Autodesk Inventor part; units mm, degrees
ref_plane "Work Plane2" through (-27.2, 5.425, 1.675) normal (1, 0, 0) x (0, 1, 0)
ref_plane "Work Plane3" through (-22.5, 37.5, -3) normal (-1, 0, 0) x (0, 0, 1)
ref_plane "YZ Plane" through (0, 0, 0) normal (1, 0, 0) x (0, 1, 0)
ref_plane "Work Plane1" through (-73.7, 19.125, 15.375) normal (-1, 0, 0) x (0, 1, 0)
sketch "Sketch1" plane through (-73.7, 19.125, 15.375) normal (-1, 0, 0) x (0, 1, 0)
  line L0 (18.375, 18.375) -> (-92.625, 18.375)
  line L1 (-92.625, 18.375) -> (-92.625, 15.375)
  line L2 (18.375, 15.375) -> (-92.625, 15.375)
  line L3 (18.375, 18.375) -> (18.375, 15.375)
  line L4 (11, 1.5) -> (11.5, 1.5)
  line L5 (11.5, 1.5) -> (11.5, -1.5)
  line L6 (11.5, -1.5) -> (11, -1.5)
  line L7 (11, -1.5) -> (11, 1.5)
  line L8 (-11.5, -1.5) -> (-12, -1.5)
  line L9 (-12, -1.5) -> (-12, 1.5)
  line L10 (-12, 1.5) -> (-11.5, 1.5)
  line L11 (-11.5, 1.5) -> (-11.5, -1.5)
  circle A0 centre (0, 0) radius 5
  circle A1 centre (0, 0) radius 13.7
  line L12 (18.375, 15.375) -> (-18.1, 15.375)
  line L13 (-18.1, 15.375) -> (-18.1, -4)
  line L14 (-18.1, -4) -> (18.375, -4)
  line L15 (18.375, -4) -> (18.375, 15.375)
  point P0 (-19.125, 15.375)
  point P1 (-13.7, 0)
  point P2 (13.7, 0)
  point P3 (-18.1, 15.375)
  point P4 (-13.1031, -4)
  point P5 (13.1031, -4)
  dimension "d0" = 4
  dimension "d2" = 15.375
  dimension "d3" = 15.375
  dimension "d4" = 4.675
  dimension "d5" = 4.4
ref_plane "Work Plane2" through (-27.2, 5.425, 1.675) normal (1, 0, 0) x (0, 1, 0)
extrude "Extrusion1" add sketch "Sketch1" against normal up to surface (46.5 mm away) contours L15 L14 A1 L13 L2
sketch "Sketch2" plane through (-27.2, 19.125, 15.375) normal (1, 0, 0) x (0, 0, -1)
  circle A0 centre (0, -8) radius 1.0564
  circle A1 centre (0, 8) radius 1.0564
  circle A2 centre (0, 0) radius 5
  circle A3 centre (0, 0) radius 13.7
  line L0 (18.375, 18.375) -> (18.375, -91.625)
  arc A4 (1.3629, -5.6821) -> (1.478, -3.5703) centre (-3.2424, -4.3721) ccw
  arc A5 (1.478, -3.5703) -> (2.0183, -3.2951) centre (0, 0) ccw
  arc A6 (2.0183, -3.2951) -> (3.794, -4.444) centre (5.443, 0.0511) ccw
  arc A7 (3.794, -4.444) -> (4.4425, -3.7958) centre (0, 0) ccw
  arc A8 (4.4425, -3.7958) -> (3.2943, -2.0197) centre (-0.0533, -5.443) ccw
  arc A9 (3.2943, -2.0197) -> (3.5697, -1.4795) centre (0, 0) ccw
  arc A10 (3.5697, -1.4795) -> (5.6815, -1.3652) centre (4.3734, 3.2407) ccw
  arc A11 (5.6815, -1.3652) -> (5.8252, -0.4596) centre (0, 0) ccw
  arc A12 (5.8252, -0.4596) -> (3.8523, 0.3024) centre (3.1561, -4.4348) ccw
  arc A13 (3.8523, 0.3024) -> (3.7575, 0.9013) centre (0, 0) ccw
  arc A14 (3.7575, 0.9013) -> (5.3989, 2.235) centre (1.6334, 5.1924) ccw
  arc A15 (5.3989, 2.235) -> (4.9828, 3.0521) centre (0, 0) ccw
  arc A16 (4.9828, 3.0521) -> (2.9388, 2.5089) centre (5.1601, -1.7327) ccw
  arc A17 (2.9388, 2.5089) -> (2.5101, 2.9378) centre (0, 0) ccw
  arc A18 (2.5101, 2.9378) -> (3.0541, 4.9816) centre (-1.7306, 5.1608) ccw
  arc A19 (3.0541, 4.9816) -> (2.2372, 5.398) centre (0, 0) ccw
  arc A20 (2.2372, 5.398) -> (0.9028, 3.7572) centre (5.193, 1.6313) ccw
  arc A21 (0.9028, 3.7572) -> (0.304, 3.8521) centre (0, 0) ccw
  arc A22 (0.304, 3.8521) -> (-0.4573, 5.8253) centre (-4.4335, 3.1579) ccw
  arc A23 (-0.4573, 5.8253) -> (-1.3629, 5.6821) centre (0, 0) ccw
  arc A24 (-1.3629, 5.6821) -> (-1.478, 3.5703) centre (3.2424, 4.3721) ccw
  arc A25 (-1.478, 3.5703) -> (-2.0183, 3.2951) centre (0, 0) ccw
  arc A26 (-2.0183, 3.2951) -> (-3.794, 4.444) centre (-5.443, -0.0511) ccw
  arc A27 (-3.794, 4.444) -> (-4.4425, 3.7958) centre (0, 0) ccw
  arc A28 (-4.4425, 3.7958) -> (-3.2943, 2.0197) centre (0.0533, 5.443) ccw
  arc A29 (-3.2943, 2.0197) -> (-3.5697, 1.4795) centre (0, 0) ccw
  arc A30 (-3.5697, 1.4795) -> (-5.6815, 1.3652) centre (-4.3734, -3.2407) ccw
  arc A31 (-5.6815, 1.3652) -> (-5.8252, 0.4596) centre (0, 0) ccw
  arc A32 (-5.8252, 0.4596) -> (-3.8523, -0.3024) centre (-3.1561, 4.4348) ccw
  arc A33 (-3.8523, -0.3024) -> (-3.7575, -0.9013) centre (0, 0) ccw
  arc A34 (-3.7575, -0.9013) -> (-5.3989, -2.235) centre (-1.6334, -5.1924) ccw
  arc A35 (-5.3989, -2.235) -> (-4.9828, -3.0521) centre (0, 0) ccw
  arc A36 (-4.9828, -3.0521) -> (-2.9388, -2.5089) centre (-5.1601, 1.7327) ccw
  arc A37 (-2.9388, -2.5089) -> (-2.5101, -2.9378) centre (0, 0) ccw
  arc A38 (-2.5101, -2.9378) -> (-3.0541, -4.9816) centre (1.7306, -5.1608) ccw
  arc A39 (-3.0541, -4.9816) -> (-2.2372, -5.398) centre (0, 0) ccw
  arc A40 (-2.2372, -5.398) -> (-0.9028, -3.7572) centre (-5.193, -1.6313) ccw
  arc A41 (-0.9028, -3.7572) -> (-0.304, -3.8521) centre (0, 0) ccw
  arc A42 (-0.304, -3.8521) -> (0.4573, -5.8253) centre (4.4335, -3.1579) ccw
  arc A43 (0.4573, -5.8253) -> (1.3629, -5.6821) centre (0, 0) ccw
  line L1 (15.375, -18.1) -> (-4, -18.1)
  line L2 (15.375, 18.375) -> (15.375, -18.1)
  line L3 (-4, 18.375) -> (15.375, 18.375)
  line L4 (-4, 13.1031) -> (-4, 18.375)
  arc A44 (-4, -13.1031) -> (-4, 13.1031) centre (0, 0) ccw
  line L5 (-4, -18.1) -> (-4, -13.1031)
  line L6 (-4, -18.1) -> (-4, -13.1031)
  line L7 (15.375, 18.375) -> (15.375, -18.1)
  line L8 (-4, -18.1) -> (15.375, -18.1)
  line L9 (15.375, -18.1) -> (15.375, 18.375)
  line L10 (15.375, 18.375) -> (-4, 18.375)
  line L11 (-4, 18.375) -> (-4, -18.1)
  circle A45 centre (0, -8) radius 1.0564
  circle A46 centre (0, 8) radius 1.0564
  arc A47 (6.0944, -1.7595) -> (6.3397, -0.2124) centre (0, 0) ccw
  arc A48 (3.9887, -2.0334) -> (6.0944, -1.7595) centre (4.3734, 3.2407) ccw
  arc A49 (5.0041, -3.8982) -> (3.9887, -2.0334) centre (-0.0533, -5.443) ccw
  arc A50 (3.8962, -5.0057) -> (5.0041, -3.8982) centre (0, 0) ccw
  arc A51 (2.0318, -3.9896) -> (3.8962, -5.0057) centre (5.443, 0.0511) ccw
  arc A52 (1.7571, -6.0951) -> (2.0318, -3.9896) centre (-3.2424, -4.3721) ccw
  arc A53 (0.2098, -6.3398) -> (1.7571, -6.0951) centre (0, 0) ccw
  arc A54 (-0.7013, -4.4219) -> (0.2098, -6.3398) centre (4.4335, -3.1579) ccw
  arc A55 (-2.1611, -5.9638) -> (-0.7013, -4.4219) centre (-5.193, -1.6313) ccw
  arc A56 (-3.5567, -5.2523) -> (-2.1611, -5.9638) centre (0, 0) ccw
  arc A57 (-3.1665, -3.1652) -> (-3.5567, -5.2523) centre (1.7306, -5.1608) ccw
  arc A58 (-5.2538, -3.5545) -> (-3.1665, -3.1652) centre (-5.1601, 1.7327) ccw
  arc A59 (-5.9647, -2.1587) -> (-5.2538, -3.5545) centre (0, 0) ccw
  arc A60 (-4.4222, -0.6995) -> (-5.9647, -2.1587) centre (-1.6334, -5.1924) ccw
  arc A61 (-6.3397, 0.2124) -> (-4.4222, -0.6995) centre (-3.1561, 4.4348) ccw
  arc A62 (-6.0944, 1.7595) -> (-6.3397, 0.2124) centre (0, 0) ccw
  arc A63 (-3.9887, 2.0334) -> (-6.0944, 1.7595) centre (-4.3734, -3.2407) ccw
  arc A64 (-5.0041, 3.8982) -> (-3.9887, 2.0334) centre (0.0533, 5.443) ccw
  arc A65 (-3.8962, 5.0057) -> (-5.0041, 3.8982) centre (0, 0) ccw
  arc A66 (-2.0318, 3.9896) -> (-3.8962, 5.0057) centre (-5.443, -0.0511) ccw
  arc A67 (-1.7571, 6.0951) -> (-2.0318, 3.9896) centre (3.2424, 4.3721) ccw
  arc A68 (-0.2098, 6.3398) -> (-1.7571, 6.0951) centre (0, 0) ccw
  arc A69 (0.7013, 4.4219) -> (-0.2098, 6.3398) centre (-4.4335, 3.1579) ccw
  arc A70 (2.1611, 5.9638) -> (0.7013, 4.4219) centre (5.193, 1.6313) ccw
  arc A71 (3.5567, 5.2523) -> (2.1611, 5.9638) centre (0, 0) ccw
  arc A72 (3.1665, 3.1652) -> (3.5567, 5.2523) centre (-1.7306, 5.1608) ccw
  arc A73 (5.2538, 3.5545) -> (3.1665, 3.1652) centre (5.1601, -1.7327) ccw
  arc A74 (5.9647, 2.1587) -> (5.2538, 3.5545) centre (0, 0) ccw
  arc A75 (4.4222, 0.6995) -> (5.9647, 2.1587) centre (1.6334, 5.1924) ccw
  arc A76 (6.3397, -0.2124) -> (4.4222, 0.6995) centre (3.1561, -4.4348) ccw
  circle A77 centre (0, 0) radius 6.3433
  point P0 (15.375, -19.125)
  point P1 (-4, 13.1031)
  point P2 (-4, 4.9231)
  point P3 (-3.8962, 5.0057)
  point P4 (-1.7571, 6.0951)
  point P5 (-0.2098, 6.3398)
  point P6 (2.1611, 5.9638)
  point P7 (3.5567, 5.2523)
  point P8 (5.2538, 3.5545)
  point P9 (5.9647, 2.1587)
  point P10 (6.3397, -0.2124)
  point P11 (5.0041, -3.8982)
  point P12 (3.8962, -5.0057)
  point P13 (1.7571, -6.0951)
  point P14 (0.2098, -6.3398)
  point P15 (-2.1611, -5.9638)
  point P16 (-3.5567, -5.2523)
  point P17 (-4, -4.9231)
  dimension "d8" = 0.5
ref_plane "Work Plane3" through (-22.5, 37.5, -3) normal (-1, 0, 0) x (0, 0, 1)
extrude "Extrusion2" add sketch "Sketch2" along normal up to surface (4.7 mm away) contours A77 A74 A71 A68 A65 L11 A3 A56 A53 A50 A47 | L4 L3 L2 L1 L5 A3
sketch "Sketch3" plane through (-73.7, 32.2281, 19.375) normal (0, 0, 1) x (1, 0, 0)
  line L0 (0, 5.2719) -> (51.2, 5.2719)
  line L1 (0, 0) -> (0, 5.2719)
  line L2 (0, 0) -> (46.5, 0)
  line L3 (46.5, 0) -> (46.5, -8.1799)
  line L4 (46.5, -8.1799) -> (51.2, -8.1799)
  line L5 (51.2, 5.2719) -> (51.2, -8.1799)
  line L6 (0, -26.2061) -> (46.5, -26.2061)
  line L7 (0, -31.2031) -> (0, -26.2061)
  line L8 (0, -31.2031) -> (51.2, -31.2031)
  line L9 (51.2, -18.0262) -> (51.2, -31.2031)
  line L10 (46.5, -18.0262) -> (51.2, -18.0262)
  line L11 (46.5, -18.0262) -> (46.5, -26.2061)
  line L12 (2.5, 2.7719) -> (48.7, 2.7719)
  line L13 (48.7, 2.7719) -> (48.7, -28.7031)
  line L14 (48.7, -28.7031) -> (2.5, -28.7031)
  line L15 (2.5, -28.7031) -> (2.5, 2.7719)
  point P0 (73.7, -32.2281)
  dimension "d11" = 2.5
  dimension "d12" = 2.5
  dimension "d13" = 2.5
  dimension "d14" = 2.5
hole "Hole1" at (-71.2, 3.525, 19.375) at (-71.2, 35, 19.375) at (-25, 35, 19.375) at (-25, 3.525, 19.375) direction (0, 0, -1) diameter 3.6 end through all counterbore diameter 11 counterbore depth 0
ref_plane "Work Plane4" through (-60.4, 19.125, 15.375) normal (-1, 0, 0) x (0, 1, 0)
sketch "Sketch4" plane through (-60.4, 19.125, 15.375) normal (-1, 0, 0) x (0, 1, 0)
  circle A0 centre (0, 0) radius 14.375
  point P0 (-19.125, 15.375)
extrude "Extrusion3" cut sketch "Sketch4" against normal blind 28.7
properties part number "motor_mount_right"
Check sheet for the modelled part. Datum: model origin and axes. Units: mm. A direction names the side the tool comes from. Round coordinates to 2 decimals unless told otherwise and drop trailing zeros. Write each loop counter-clockwise with the first axis right and the second up, starting at its lowest first coordinate (ties: lowest second). Pieces come first, ordered by that corner, then holes. Notation, with made-up numbers: (-15, 76.25) - (-8, 76.25) arc R28 ccw to (-8, 115.25) - close; hole circle Ø6 at (-32.5, -36). An arc over 180 degrees is marked (long way). Return JSON: item names as keys, results as strings.
Q1. Cross-section at D-D (x = -71.2). Record the boundary of the cut face in (y, z) (3 decimals).
Returned:
{"outline": "(1.025, 0) - (1.725, 0) - (1.725, 19.375) - (1.025, 19.375) - close; (5.325, 0) - (33.2, 0) - (33.2, 19.375) - (32.228, 19.375) arc R13.7 cw (long way) to (6.022, 19.375) - (5.325, 19.375) - close; (36.8, 0) - (37.5, 0) - (37.5, 19.375) - (36.8, 19.375) - close"}
Q2. Draft check along Z on faces 1 (the cylindrical face through (-24.88, 25.39, 16.38)), 2 (the flat face through (-46, 34, 19.375)), 3 (the flat face through (-22.5, 20, 8)). Enter one of: released by +Z, released by -Z, zero draft, split by the parting line, or undercut.
Returned:
{"face 1": "undercut", "face 2": "released by +Z", "face 3": "zero draft"}
Q3. Cross-section at B-B (x = -25). Give the number of separate pieces and of enclosed holes in the cut face, then the cut area to 3 significant figures.
Returned:
{"separate pieces": "3", "enclosed holes": "2", "area": "450 mm²"}
Q4. Access from +Z, -Z, +X, -X, +Y, -Y to the whole of each face (thin tool, end or side, straight path). Record for faces 4 (the flat face through (-48, 37.5, 10)), 5 (the cylindrical face through (-24.883, 22.013, 9.727)), 6 (the cylindrical face through (-24.88, 13.48, 12.48)), 7 (the flat face through (-60.4, 19.1, 1.3)), 8 (the cylindrical face through (-26.518, 34.032, 9.552)).
Returned:
{"face 4": "+Z, -Z, +X, -X, +Y", "face 5": "+Z, +X, -X", "face 6": "+X, -X", "face 7": "none", "face 8": "+Z, -Z"}
Q5. Scan lines: L1, parallel to X at y = 35, z = 11.5; L2, parallel to Y at x = -25, z = 8.25 (3 decimals); L3, parallel to Y at x = -25, z = 14.25 (3 decimals). Record each from-to range of solid material in increasing order. Write a range as from..to.
Returned:
{"L1": "x = -73.7..-73, -69.4..-26.8, -23.2..-22.5", "L2": "y = 1.025..1.725, 5.325..33.2, 36.8..37.5", "L3": "y = 1.025..1.725, 5.325..12.882, 25.368..33.2, 36.8..37.5"}
Q6. Cross-section at A-A (y = 35). Record the boundary of the cut face in (x, z) (3 decimals), then the cut area to 4 significant figures.
Returned:
{"outline": "(-73.7, 0) - (-73, 0) - (-73, 19.375) - (-73.7, 19.375) - close; (-69.4, 0) - (-26.8, 0) - (-26.8, 19.375) - (-69.4, 19.375) - close; (-23.2, 0) - (-22.5, 0) - (-22.5, 19.375) - (-23.2, 19.375) - close", "area": "852.5 mm²"}
Q7. Cross-section at C-C (z = 5.75). Record the boundary of the cut face in (x, y) (3 decimals).
Returned:
{"outline": "(-73.7, 1.025) - (-22.5, 1.025) - (-22.5, 37.5) - (-73.7, 37.5) - (-73.7, 28.874) - (-60.4, 28.874) - (-60.4, 29.802) - (-31.7, 29.802) - (-31.7, 28.874) - (-27.2, 28.874) - (-27.2, 9.376) - (-31.7, 9.376) - (-31.7, 8.448) - (-60.4, 8.448) - (-60.4, 9.376) - (-73.7, 9.376) - close; hole circle Ø3.6 at (-71.2, 3.525); hole circle Ø3.6 at (-71.2, 35); hole circle Ø3.6 at (-25, 3.525); hole circle Ø3.6 at (-25, 35)"}
Q8. Depth check by flat-ended pin: P1, Ø5.5, axis at y = 15.5, z = 15, coming from the -X side; P2, Ø10, axis at x = -40.5, y = 30, coming from the +Z side (3 decimals). Enter the tip coordinate at first touch or a pass-through.
Returned:
{"P1": "stops at x = -27.2", "P2": "stops at z = 19.375"}
